```python
from build123d import *

# Parameters (mm, degrees)
RESSALTO_EXTRUS_O1_DEPTH         = 1.5
RESSALTO_EXTRUS_O2_START         = 22
ESBO_O2_R                        = 2.5
RESSALTO_EXTRUS_O2_DEPTH         = 22
RESSALTO_EXTRUS_O3_START         = 22
ESBO_O3_R                        = 2.5
RESSALTO_EXTRUS_O3_DEPTH         = 22
FURO_DE_DI_METRO_3_0_3_1_D       = 3
FURO_DE_DI_METRO_20_0_20_1_D     = 20
FURO_DE_DI_METRO_20_0_20_1_DEPTH = 23.5
ESBO_O8_R                        = 2.5
CORTE_EXTRUS_O1_DEPTH            = 13


with BuildPart() as part:
    # Esboço1 → Ressalto-extrusão1 (new body)
    with BuildSketch(Plane(origin=(0, 0, 0), x_dir=(-1, 0, 0), z_dir=(0, 0, -1))):
        with BuildLine():
            Line((13.774977314, -2.5), (19.85, -2.5))
            ThreePointArc((19.85, -2.5), (22.35, 0), (19.85, 2.5))
            Line((19.85, 2.5), (13.774977314, 2.5))
            ThreePointArc((13.774977314, 2.5), (0, 14), (-13.774977314, 2.5))
            Line((-13.774977314, 2.5), (-19.85, 2.5))
            ThreePointArc((-19.85, 2.5), (-22.35, 0), (-19.85, -2.5))
            Line((-19.85, -2.5), (-13.774977314, -2.5))
            ThreePointArc((-13.774977314, -2.5), (0, -14), (13.774977314, -2.5))
        make_face()
    extrude(amount=-RESSALTO_EXTRUS_O1_DEPTH)

    # Esboço2 → Ressalto-extrusão2 (add)
    with BuildSketch(Plane(origin=(0, 0, 0), x_dir=(-1, 0, 0), z_dir=(0, 0, -1)).offset(RESSALTO_EXTRUS_O2_START)):
        with Locations((-19.85, 0)):
            Circle(ESBO_O2_R)
    extrude(amount=-RESSALTO_EXTRUS_O2_DEPTH)

    # Esboço3 → Ressalto-extrusão3 (add)
    with BuildSketch(Plane(origin=(0, 0, 0), x_dir=(-1, 0, 0), z_dir=(0, 0, -1)).offset(RESSALTO_EXTRUS_O3_START)):
        with Locations((19.85, 0)):
            Circle(ESBO_O3_R)
    extrude(amount=-RESSALTO_EXTRUS_O3_DEPTH)

    # Furo de diâmetro Ø3.0 (3)1 (through all)
    with Locations(Plane(origin=(0, 0, -22), x_dir=(-1, 0, 0), z_dir=(0, 0, -1))):
        with Locations((-19.85, 0), (19.85, 0)):
            Hole(FURO_DE_DI_METRO_3_0_3_1_D / 2)

    # Furo de diâmetro Ø20.0 (20)1
    with Locations(Plane.XY.offset(1.5)):
        with Locations((0, 0)):
            Hole(FURO_DE_DI_METRO_20_0_20_1_D / 2, depth=FURO_DE_DI_METRO_20_0_20_1_DEPTH)

    # Esboço8 → Corte-extrusão1 (cut)
    with BuildSketch(Plane(origin=(0, 0, -22), x_dir=(-1, 0, 0), z_dir=(0, 0, -1))):
        with Locations((19.85, 0)):
            Circle(ESBO_O8_R)
        with Locations((-19.85, 0)):
            Circle(ESBO_O8_R)
    extrude(amount=-CORTE_EXTRUS_O1_DEPTH, mode=Mode.SUBTRACT)


solid = part.part
```
Build history of the part. All positions in model axes, mm. A direction names the side the tool comes from. Round coordinates to 2 decimals unless told otherwise and drop trailing zeros. Order: outer loops, then holes, each group sorted by start corner. A loop starts at its lowest first (then second) coordinate and runs counter-clockwise, first axis right, second up. Notation, with made-up numbers: (-40, 50.5) -> (16, 50.5) arc R15 cw to (16, 55.5) -> close; hole circle Ø2 at (2.25, -30.75). An arc over 180 degrees is marked (long way). Answer in a Markdown table with one row per item.
1) Wall check: L1, parallel to Y at x = -19.85, z = -6.25; L2, parallel to Y at x = -14, z = 1.25; L3, parallel to Z at x = 14, y = -1.5. Give the ranges that are in metal, low to high.
Values:
| item | result |
|---|---|
| L1 | -2.5 to -1.5, 1.5 to 2.5 |
| L2 | -2.5 to 2.5 |
| L3 | 0 to 1.5 |
2) Pin check, flat tips, straight feed: P1, Ø3, axis at y = 10, z = -0.5, coming from the -X side; P2, Ø4, axis at x = 13.5, z = -4.5, coming from the +Y side; P3, Ø1, axis at x = -15, z = 0, coming from the -Y side; P4, Ø10, axis at x = -14.5, y = -1.5, coming from the -Z side. Stop position of each tip, or through.
Values:
| item | result |
|---|---|
| P1 | x = -11.06 |
| P2 | through |
| P3 | y = -2.5 |
| P4 | z = -9 |
3) Mould opens along X. For faces 6 (the cylindrical face through (0, 14, 1)), 7 (the flat face through (10, 2, 1.5)), 8 (the cylindrical face through (22.348, 0.11, -3.823)) say: released by +X, released by -X, zero draft, split by the parting line, or undercut.
Values:
| item | result |
|---|---|
| face 6 | split by the parting line |
| face 7 | zero draft |
| face 8 | undercut |
4) Band-saw the part on A-A on z = -6. Give the cut face in (x, y).
Values:
| item | result |
|---|---|
| outline | circle Ø5 at (-19.85, 0); circle Ø5 at (19.85, 0); hole circle Ø3 at (-19.85, 0); hole circle Ø3 at (19.85, 0) |
5) Band-saw the part on D-D on x = -15.5. Give the cut face in (y, z).
Values:
| item | result |
|---|---|
| outline | (-2.5, 0) -> (2.5, 0) -> (2.5, 1.5) -> (-2.5, 1.5) -> close |
6) Band-saw the part on C-C on x = 0. Give the cut face in (y, z), and give its area (3 significant figures).
Values:
| item | result |
|---|---|
| outline | (-14, 0) -> (-10, 0) -> (-10, 1.5) -> (-14, 1.5) -> close; (10, 0) -> (14, 0) -> (14, 1.5) -> (10, 1.5) -> close |
| area | 12.0 mm2 |
7) Which spindle directions (+Z, -Z, +X, -X, +Y, -Y) get a long thin tool onto all of the face, cutting with end or side? Do faces 1 (the flat face through (-17, 2.5, 1)), 2 (the flat face through (17, 2.5, 1)), 3 (the flat face through (20, -2, -9)), 4 (the flat face through (17, -2.5, 1)), 5 (the flat face through (-17, -2.5, 1)). Say none if no direction does.
Values:
| item | result |
|---|---|
| face 1 | +Z, -Z, -X, +Y |
| face 2 | +Z, -Z, +X, +Y |
| face 3 | -Z, +X, -X, +Y, -Y |
| face 4 | +Z, -Z, +X, -Y |
| face 5 | +Z, -Z, -X, -Y |
8) Band-saw the part on B-B on y = -4. Give the cut face in (x, z), and give its area (3 significant figures).
Values:
| item | result |
|---|---|
| outline | (-13.42, 0) -> (-9.17, 0) -> (-9.17, 1.5) -> (-13.42, 1.5) -> close; (9.17, 0) -> (13.42, 0) -> (13.42, 1.5) -> (9.17, 1.5) -> close |
| area | 12.8 mm2 |
